Autodesk Inventor part; units mm, degrees
ref_plane "YZ Plane" through (0, 0, 0) normal (1, 0, 0) x (0, 1, 0)
ref_plane "XZ Plane" through (0, 0, 0) normal (0, 1, 0) x (-1, 0, 0)
ref_plane "XY Plane" through (0, 0, 0) normal (0, 0, 1) x (1, 0, 0)
sketch "スケッチ1" plane through (0, 0, 0) normal (0, 1, 0) x (-1, 0, 0)
  line L0 (0, 0) -> (0, -40)
  line L1 (0, -40) -> (-23.7735, -40)
  line L2 (-23.7735, -40) -> (-54.0844, -22.5)
  line L3 (0, -30) -> (-18, -30)
  line L4 (-18, -30) -> (-38, -18.453)
  line L5 (-28, -24.2265) -> (-28, 11.9512)
  line L6 (-18, -30) -> (-23.7735, -40)
  line L7 (-18.7735, -31.3397) -> (-20.74, -30.2044)
  line L8 (-20.74, -30.2044) -> (-58.951, -8.1433)
  line L9 (-33.7735, -34.2265) -> (-30.4735, -28.5107)
  line L10 (-30.4735, -28.5107) -> (-47.5342, -18.6607)
  line L11 (-47.5342, -18.6607) -> (-50.8342, -24.3765)
  line L12 (-50.8342, -24.3765) -> (-33.7735, -34.2265)
  line L13 (-30.4735, -28.5107) -> (-28, -24.2265)
  line L14 (-24.6395, -39.5) -> (-19.5508, -30.686)
  line L15 (-54.0844, -22.5) -> (-49.0844, -13.8397)
  point P0 (-19.6395, -30.8397)
  dimension "d0" = 40
  dimension "d1" = 30
  dimension "d2" = 18
  dimension "d3" = 30
  dimension "d4" = 38
  dimension "d5" = 10
  dimension "d6" = 10
  dimension "d7" = 19.7
  dimension "d8" = 6.6
  dimension "d9" = 1
  dimension "d10" = 35
extrude "押し出し1" add sketch "スケッチ1" along normal blind 15 contours L2 L9 L13 L8 L7 L14 | L13 L10 L11 L2 L15 L8
sketch "スケッチ2" plane through (0, 0, 0) normal (0, -1, 0) x (1, 0, 0)
  line L0 (30.4735, -28.5107) -> (33.7735, -34.2265)
  line L1 (47.5342, -18.6607) -> (30.4735, -28.5107)
  line L2 (50.8342, -24.3765) -> (47.5342, -18.6607)
  line L3 (54.0844, -22.5) -> (50.8342, -24.3765)
  line L4 (49.0844, -13.8397) -> (54.0844, -22.5)
  line L5 (19.6395, -30.8397) -> (49.0844, -13.8397)
  line L6 (24.6395, -39.5) -> (19.6395, -30.8397)
  line L7 (33.7735, -34.2265) -> (24.6395, -39.5)
  line L8 (50.8342, -24.3765) -> (33.7735, -34.2265)
  point P0 (0, 0)
extrude "押し出し2" add sketch "スケッチ2" against normal blind 1
sketch "スケッチ3" plane through (30.4735, 1, -28.5107) normal (0.5, 0, -0.8660254) x (-0.8660254, 0, -0.5)
  line L0 (-19.7, 0) -> (0, 0)
  line L1 (-19.7, 14) -> (0, 14)
  line L2 (-9.85, 14) -> (-9.85, 0)
  line L3 (-19.7, 0) -> (0, 0)
  circle A0 centre (-14.6, 7.9) radius 0.85
  circle A1 centre (-5.1, 7.9) radius 0.85
  point P0 (12.1355, -1)
  dimension "d16" = 1.7
  dimension "d17" = 9.5
  dimension "d18" = 7.9
extrude "押し出し3" cut sketch "スケッチ3" against normal through all
sketch "スケッチ4" plane through (0, 0, 0) normal (0, -1, 0) x (1, 0, 0)
  circle A0 centre (50.5, 0) radius 1.35
  circle A1 centre (50.5, 0) radius 12.5
  line L0 (49.0844, -13.8397) -> (54.0844, -22.5)
  line L1 (49.0844, -13.8397) -> (54.0844, -22.5)
  line L2 (54.0844, -22.5) -> (74.7158, -10.5885)
  line L3 (74.7158, -10.5885) -> (69.7158, -1.9282)
  line L4 (69.7158, -1.9282) -> (49.0844, -13.8397)
  line L5 (74.7158, -10.5885) -> (86.6025, 10)
  circle A2 centre (71.4838, 0.8246) radius 1.5
  circle A3 centre (71.4838, 0.8246) radius 12.5
  point P0 (0, 0)
  point P1 (60.8076, -7.0714)
  point P2 (51.4702, -12.4623)
  point P3 (72.3273, -6.4515)
  point P4 (61.4867, -6.6793)
  point P5 (72.9912, -11.5842)
  dimension "d21" = 25
  dimension "d24" = 25
extrude "押し出し4" add sketch "スケッチ4" against normal up to surface (15 mm away) contours L4 A1 | A1 L4 A3 L2 L0
sketch "スケッチ5" plane through (0, 15, 0) normal (0, 1, 0) x (1, 0, 0)
  line L0 (56.7805, 18.4608) -> (59.6305, 16.8153)
  line L1 (59.6305, 16.8153) -> (59.6305, 13.5244)
  line L2 (59.6305, 13.5244) -> (56.7805, 11.879)
  line L3 (56.7805, 11.879) -> (53.9305, 13.5244)
  line L4 (53.9305, 13.5244) -> (53.9305, 16.8153)
  line L5 (53.9305, 16.8153) -> (56.7805, 18.4608)
  line L6 (26.4697, 35.9608) -> (29.3197, 34.3153)
  line L7 (29.3197, 34.3153) -> (29.3197, 31.0244)
  line L8 (29.3197, 31.0244) -> (26.4697, 29.379)
  line L9 (26.4697, 29.379) -> (23.6197, 31.0244)
  line L10 (23.6197, 31.0244) -> (23.6197, 34.3153)
  line L11 (23.6197, 34.3153) -> (26.4697, 35.9608)
  line L12 (19.6395, 30.8397) -> (61.4867, 6.6793)
  line L13 (24.6395, 39.5) -> (19.6395, 30.8397)
  circle A0 centre (56.7805, 15.1699) radius 1.6
  circle A1 centre (26.4697, 32.6699) radius 1.6
  line L14 (23.8895, 39.933) -> (74.5998, 10.6554)
  line L15 (59.6305, 13.5244) -> (62.1305, 17.8546)
  line L16 (53.9305, 16.8153) -> (56.4305, 21.1454)
  line L17 (29.3197, 31.0244) -> (31.8197, 35.3546)
  line L18 (23.6197, 34.3153) -> (26.1197, 38.6454)
  point P0 (0, 0)
  dimension "d25" = 5.7
  dimension "d26" = 5
  dimension "d27" = 5
  dimension "d28" = 40
  dimension "d29" = 3.2
extrude "押し出し5" cut sketch "スケッチ5" against normal blind 10 contours L5 L16 L14 L15 L1 L0 | L0 L1 L2 L3 L4 L5 | L11 L18 L14 L17 L7 L6 | L6 L7 L8 L9 L10 L11 | A0 | A1
extrude "押し出し6" cut sketch "スケッチ5" against normal through all contours A0 | A1
sketch "スケッチ6" plane through (0, 0, 0) normal (0, -1, 0) x (1, 0, 0)
  arc A0 (28.6476, -35.6197) -> (24.5492, -37.9938) centre (27, -37.5) ccw
  arc A1 (23.7735, -40) -> (24.5492, -37.9938) centre (22.5886, -38.3888) ccw
  arc A2 (28.6476, -35.6197) -> (30.9657, -35.8476) centre (29.9657, -34.1155) ccw
  arc A3 (72.5905, -10.2571) -> (68.4853, -12.6194) centre (70.9375, -12.1327) ccw
  arc A4 (67.5236, -14.7409) -> (68.4853, -12.6194) centre (66.5236, -13.0088) ccw
  circle A5 centre (26.4697, -32.6699) radius 1.6
  circle A6 centre (56.7805, -15.1699) radius 1.6
  line L0 (24.6395, -39.5) -> (72.9912, -11.5842)
  arc A7 (61.4867, -6.6793) -> (72.9912, -11.5842) centre (71.4838, 0.8246) ccw
  line L1 (19.6395, -30.8397) -> (61.4867, -6.6793)
  line L2 (24.6395, -39.5) -> (19.6395, -30.8397)
  point P0 (0, 0)
  point P1 (24.4378, -39.1507)
  point P2 (68.5695, -11.3309)
extrude "押し出し7" cut sketch "スケッチ6" against normal through all contours A2 L0 L2 A1 A0 | A4 A3 A7 L0
extrude "押し出し8" add sketch "スケッチ5" against normal blind 7
properties part number "limit_setter_under"
Work out the finished part from the listing and answer in its coordinate system (mm). A direction names the side the tool comes from. Give positions to 0.01 mm unless a question says otherwise; leave off trailing zeros. Loops run counter-clockwise (first coordinate to the right, second up) from the corner with the lowest first, then second, coordinate; pieces in that order, holes last. Notation, with made-up numbers: (10, -14.5) - (44, -14.5) arc R28 ccw to (44, 12.5) - close; hole circle Ø2 at (67, 26). An arc over 180 degrees is marked (long way). Answer in a Markdown table with one row per item.
(1) For a pull along Y with two mould halves and no side action, classify faces 1 (the face through (60.863, 6.521, -15.659)), 2 (the face through (55.182, 11.549, -15.24)), 3 (the face through (44, 0, -23)) as pulls with the +Y half, pulls with the -Y half, needs draft (parallel to the pull), parting line crosses it, or undercut.
Results list:
| item | result |
|---|---|
| face 1 | undercut |
| face 2 | needs draft |
| face 3 | pulls with the -Y half |
(2) Section C-C (x = 59) is taken. Give the vertices of the cut face in (y, z).
Results list:
| item | result |
|---|---|
| outline | (0, -19.66) - (5, -19.66) - (5, -13.16) - (8, -13.16) - (8, -19.66) - (15, -19.66) - (15, -8.11) - (0, -8.11) - close |
(3) Section D-D (z = -27) is taken. Give the vertices of the cut face in (x, y), and give its area (3 significant figures).
Results list:
| item | result |
|---|---|
| outline | (26.29, 0) - (46.29, 0) - (46.29, 1) - (33.09, 1) - (33.09, 15) - (26.29, 15) - close |
| area | 115 mm² |
(4) A tool of negligible diameter and unlimited length cuts with its end or side. For faces 4 (the face through (53.93, 7, -15)), 5 (the face through (27.91, 6.52, -30.21)), 6 (the face through (25.444, 11.549, -37.475)), from which of +Z, -Z, +X, -X, +Y, -Y can it reach the whole face along a straight path? Write none if from no direction.
Results list:
| item | result |
|---|---|
| face 4 | none |
| face 5 | -Z |
| face 6 | -Z, +Y, -Y |
(5) Section A-A (x = 25.5) is taken. Give the vertices of the cut face in (y, z), and give its area (3 significant figures).
Results list:
| item | result |
|---|---|
| outline | (0, -35.5) - (5, -35.5) - (5, -33.94) - (0, -33.94) - close; (0, -31.4) - (5, -31.4) - (5, -29.94) - (8, -29.94) - (8, -31.4) - (15, -31.4) - (15, -27.46) - (0, -27.46) - close; (8, -37.57) - (15, -37.57) - (15, -33.94) - (8, -33.94) - close |
| area | 87.9 mm² |
(6) Section B-B (y = 3.25) is taken. Give the vertices of the cut face in (x, z).
Results list:
| item | result |
|---|---|
| outline | (19.64, -30.84) - (24.44, -39.15) arc R2 ccw to (24.55, -37.99) arc R2.5 cw to (28.65, -35.62) arc R2 ccw to (30.97, -35.85) - (33.77, -34.23) - (30.47, -28.51) - (47.53, -18.66) - (50.83, -24.38) - (54.08, -22.5) - (67.52, -14.74) arc R2 ccw to (68.49, -12.62) arc R2.5 cw to (68.57, -11.33) arc R12.5 cw to (61.49, -6.68) - (49.08, -13.84) - (20.74, -30.2) - close; hole circle Ø3.2 at (26.47, -32.67); hole circle Ø3.2 at (56.78, -15.17) |
(7) Consider L1, parallel to X at y = 9, z = -38; L2, parallel to Y at x = 28, z = -37.5; L3, parallel to X at y = 4.25, z = -14. Determine where each line is inside the solid, lowest interval first. Write a range as [from, to].
Results list:
| item | result |
|---|---|
| L1 | x = [23.77, 24.55], [25.75, 27.24] |
| L2 | y = [8, 15] |
| L3 | x = [48.81, 55.69], [57.87, 68.26] |
(8) Flat-ended cylindrical pins translate along their axes: pin 1 Ø2 at (y, z) = (13.5, -17) entering from -X; pin 2 Ø2.5 at (x, z) = (56.78, -15.17) entering from +Y; pin 3 Ø2.5 at (y, z) = (6, -16) entering from +X; pin 4 Ø1.5 at (y, z) = (6.5, -32) entering from +X. Find the tip coordinate at first contact, or state that the pin passes through.
Results list:
| item | result |
|---|---|
| pin 1 | stops at x = 41.88 |
| pin 2 | passes through |
| pin 3 | stops at x = 67.51 |
| pin 4 | stops at x = 32.92 |
